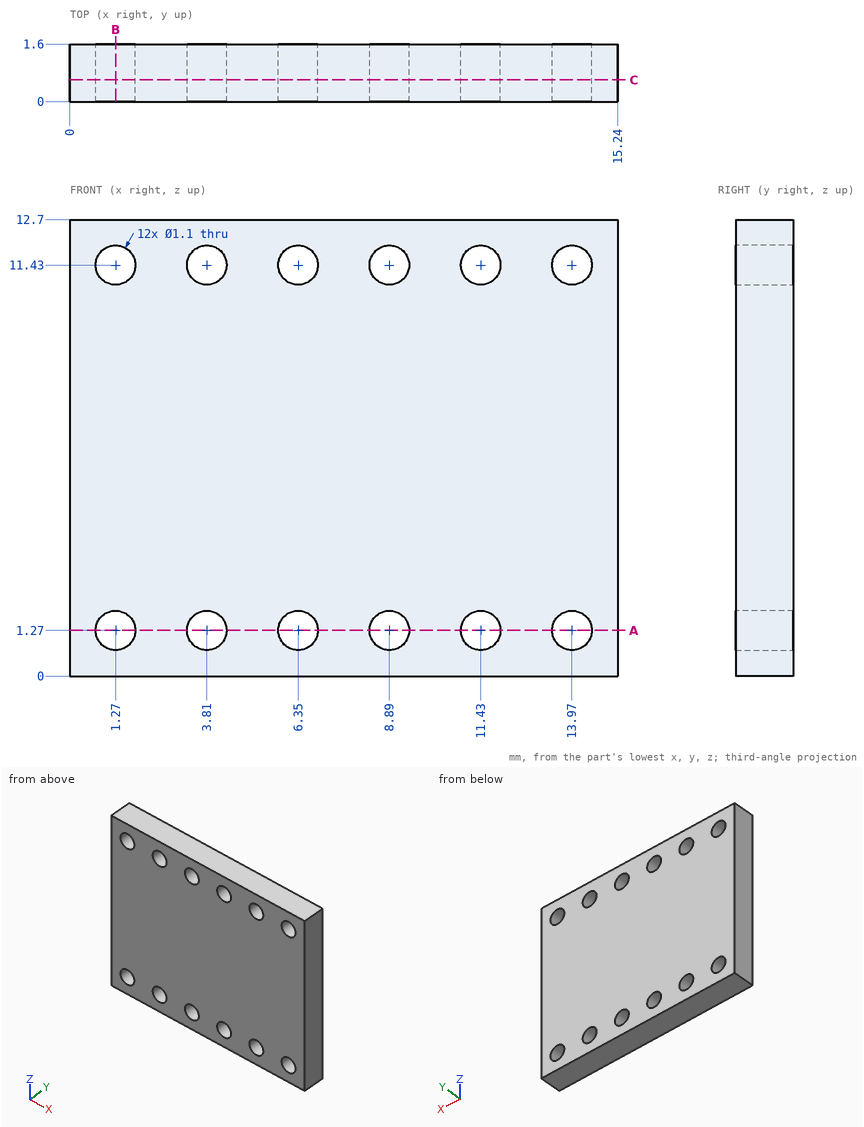
Verification items for this drawing (mm, ordinates from the low corner). Coordinates: 2 decimals unless noted, no trailing zeros. Order: outer loops, then holes, each group sorted by start corner. A loop starts at its lowest first (then second) coordinate and runs counter-clockwise, first axis right, second up. Notation, with made-up numbers: M 44,9 L 53,9 A24 cw 53,36 Z; hole C 29.5,7.5 d6. An arc over 180 degrees is marked long. Answer as a JSON object with one key per item and string values.
Q1. Scan lines: line 1 (Z direction, x = 6.5, y = 1.3); line 2 (Z direction, x = 14.25, y = 1.45). Record each from-to range of solid material in increasing order.
Results are:
{"line 1": "z = 0 to 0.74, 1.8 to 10.9, 11.96 to 12.7", "line 2": "z = 0 to 0.8, 1.74 to 10.96, 11.9 to 12.7"}
Q2. Cross-section at A-A on z = 1.27. Record the cut outline in (x, y).
Results are:
{"outline": "M 0,0 L 0.72,0 L 0.72,1.6 L 0,1.6 Z; M 1.82,0 L 3.26,0 L 3.26,1.6 L 1.82,1.6 Z; M 4.36,0 L 5.8,0 L 5.8,1.6 L 4.36,1.6 Z; M 6.9,0 L 8.34,0 L 8.34,1.6 L 6.9,1.6 Z; M 9.44,0 L 10.88,0 L 10.88,1.6 L 9.44,1.6 Z; M 11.98,0 L 13.42,0 L 13.42,1.6 L 11.98,1.6 Z; M 14.52,0 L 15.24,0 L 15.24,1.6 L 14.52,1.6 Z"}
Q3. Depth check by flat-ended pin: pin 1 Ø1.3 at (x, z) = (11.43, 11.43) entering from +Y. Enter the tip coordinate at first touch or a pass-through.
Results are:
{"pin 1": "stops at y = 1.6"}
Q4. Cross-section at B-B on x = 1.27. Record the cut outline in (y, z).
Results are:
{"outline": "M 0,0 L 1.6,0 L 1.6,0.72 L 0,0.72 Z; M 0,1.82 L 1.6,1.82 L 1.6,10.88 L 0,10.88 Z; M 0,11.98 L 1.6,11.98 L 1.6,12.7 L 0,12.7 Z"}
Q5. Cross-section at C-C on y = 0.6. Give the number of separate pieces and of enclosed holes in the cut face, and give its area (3 significant figures).
Results are:
{"separate pieces": "1", "enclosed holes": "12", "area": "182 mm²"}
